Part model, mm, in its own coordinate system. Face numbers are marked on the shaded views. Give positions to 0.01 mm unless a question says otherwise; leave off trailing zeros. Order: outer loops, then holes, each group sorted by start corner. A loop starts at its lowest first (then second) coordinate and runs counter-clockwise, first axis right, second up. Notation, with made-up numbers: (77, 70) - (94, 70) arc R35 cw to (94, 107) - close; hole circle Ø6 at (39, 49.5). An arc over 180 degrees is marked (long way). Use one line per item in the form item = value. Start each with the question number.
1. Band-saw the part on A-A, the plane y = 2.25. List the corners of the cut face in (x, z).
2. Drill centre lines: line 1 (X direction, y = 9.25, z = 0); line 2 (Z direction, x = 1.25, y = 6.75); line 3 (X direction, y = 7, z = -0.5). Where is each one in solid material? Low to high.
3. Pin check, flat tips, straight feed: P1, Ø3, axis at x = 0.5, y = 2, coming from the -Z side; P2, Ø5, axis at x = -2.5, y = 7, coming from the +Z side; P3, Ø4, axis at y = 6, z = 1.5, coming from the -X side. Stop position of each tip, or through.
4. Pull direction Z, two halves, no side cores. Call the marked faces 1, 2 and 3: +Z half, -Z half, draft (parallel to the pull), parting line (faces both ways), or undercut.
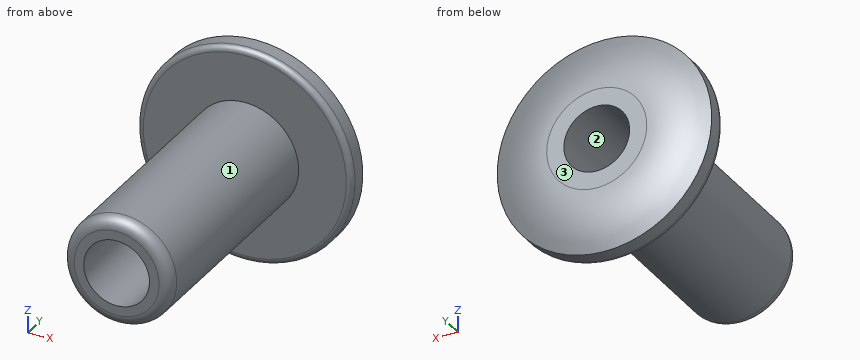
from build123d import *

# Parameters (mm, degrees)
FILLET1_R = 0.508


with BuildPart() as part:
    # Sketch1 → Revolve1 (revolve)
    with BuildSketch(Plane.XY, mode=Mode.PRIVATE) as revolve1_sk:
        with BuildLine():
            Line((-1.4605, 0), (-1.4605, 12.065))
            Line((-1.4605, 12.065), (-2.2225, 12.065))
            ThreePointArc((-2.2225, 12.065), (-3.531586036, 11.903844145), (-4.7625, 11.43))
            Line((-4.7625, 11.43), (-4.7625, 10.795))
            ThreePointArc((-4.7625, 10.795), (-4.688105122, 10.615394878), (-4.5085, 10.541))
            Line((-4.5085, 10.541), (-2.39395, 10.541))
            Line((-2.39395, 10.541), (-2.39395, 0))
            Line((-2.39395, 0), (-1.4605, 0))
        make_face()
    revolve(revolve1_sk.sketch.rotate(Axis((0, 0, 0), (0, 1, 0)), 270), axis=Axis((0, 0, 0), (0, 1, 0)))

    # Fillet1
    fillet1_edges = [part.edges().sort_by_distance(p)[0] for p in [
        (0, 0, 2.39395),
    ]]
    fillet(fillet1_edges, radius=FILLET1_R)


solid = part.part
From the geometry:
q1.outline = circle Ø4.79 at (0, 0); hole circle Ø2.92 at (0, 0)
q2.line_1 = -2.39 to -1.46, 1.46 to 2.39
q2.line_2 = -2.04 to -0.76, 0.76 to 2.04
q2.line_3 = -2.34 to -1.37, 1.37 to 2.34
q3.P1 = -2.39
q3.P2 = 2.39
q3.P3 = -2.39
q4.face_1 = parting line
q4.face_2 = undercut
q4.face_3 = draft
